Here's the drawing with two shaded views (mm, measured from the low corner). I have some questions. Round coordinates to 2 decimals unless told otherwise and drop trailing zeros. Order: outer loops, then holes, each group sorted by start corner. A loop starts at its lowest first (then second) coordinate and runs counter-clockwise, first axis right, second up. Notation, with made-up numbers: (-30.5, 29) -> (6.5, 29) arc R25 cw to (6.5, 54) -> close; hole circle Ø5 at (31.5, 27). An arc over 180 degrees is marked (long way). One line per question, with ' | ' between items.
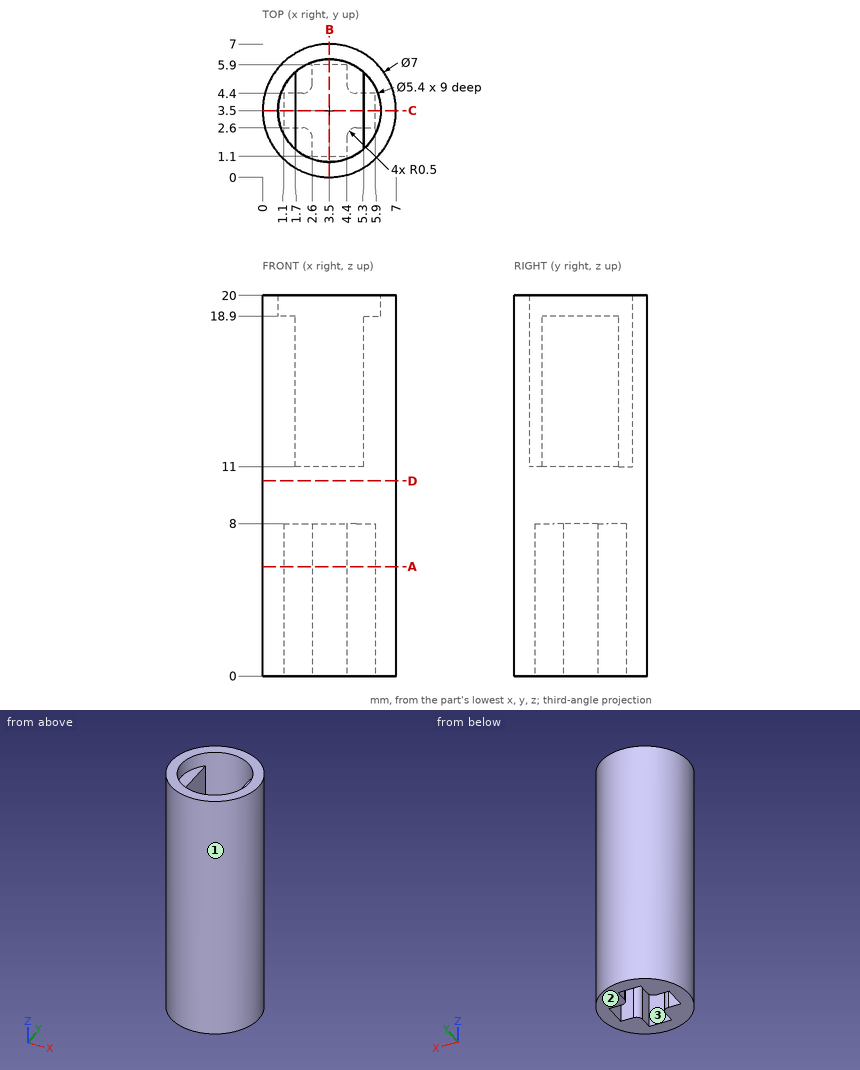
1. I want a section at B-B on x = 3.5. List the corners of the cut face in (y, z) for me.
From the geometry:
outline: (0, 0) -> (1.1, 0) -> (1.1, 8) -> (5.9, 8) -> (5.9, 0) -> (7, 0) -> (7, 20) -> (6.2, 20) -> (6.2, 11) -> (0.8, 11) -> (0.8, 20) -> (0, 20) -> close
2. I want a section at C-C on y = 3.5. List the corners of the cut face in (x, z) for me, and give its area (3 significant figures).
From the geometry:
outline: (0, 0) -> (1.1, 0) -> (1.1, 8) -> (5.9, 8) -> (5.9, 0) -> (7, 0) -> (7, 20) -> (6.2, 20) -> (6.2, 18.9) -> (5.3, 18.9) -> (5.3, 11) -> (1.7, 11) -> (1.7, 18.9) -> (0.8, 18.9) -> (0.8, 20) -> (0, 20) -> close | area: 67.2 mm²
3. I want a section at D-D on z = 10.25. List the corners of the cut face in (x, y) for me.
From the geometry:
outline: circle Ø7 at (3.5, 3.5)
4. I want a section at A-A on z = 5.75. List the corners of the cut face in (x, y) for me.
From the geometry:
outline: circle Ø7 at (3.5, 3.5); hole (1.1, 2.6) -> (2.1, 2.6) arc R0.5 cw to (2.6, 2.1) -> (2.6, 1.1) -> (4.4, 1.1) -> (4.4, 2.1) arc R0.5 cw to (4.9, 2.6) -> (5.9, 2.6) -> (5.9, 4.4) -> (4.9, 4.4) arc R0.5 cw to (4.4, 4.9) -> (4.4, 5.9) -> (2.6, 5.9) -> (2.6, 4.9) arc R0.5 cw to (2.1, 4.4) -> (1.1, 4.4) -> close
5. I'm going to push flat-ended pins straight in: pin 1 (2 mm diameter, centred on x = 3.5, y = 4, fed in from +Z); pin 2 (0.8 mm diameter, centred on x = 5.5, z = 2.5, fed in from +Y); pin 3 (0.8 mm diameter, centred on y = 5, z = 6, fed in from +X); pin 4 (2 mm diameter, centred on x = 3, z = 3, fed in from -Y). Where does each tip first touch, or does it pass through?
From the geometry:
pin 1: stops at z = 11 | pin 2: stops at y = 6.61 | pin 3: stops at x = 6.82 | pin 4: stops at y = 0
6. If we mould it in two halves opening along X, with no side actions, what happens to the marked faces 1, 2 and 3? For each: pulls with the +X half, pulls with the -X half, needs draft (parallel to the pull), parting line crosses it, or undercut.
From the geometry:
face 1: parting line crosses it | face 2: needs draft | face 3: undercut
7. I need wall thicknesses on probe 1 along Y at (x, z) = (3.5, 18.5); probe 2 along Z at (x, y) = (4, 2.75); probe 3 along Y at (x, z) = (2, 17) (3 decimals). Which ranges of each line are inside material? Lowest first, please.
From the geometry:
probe 1: y = 0 to 0.8, 6.2 to 7 | probe 2: z = 8 to 11 | probe 3: y = 0.338 to 1.255, 5.745 to 6.662
